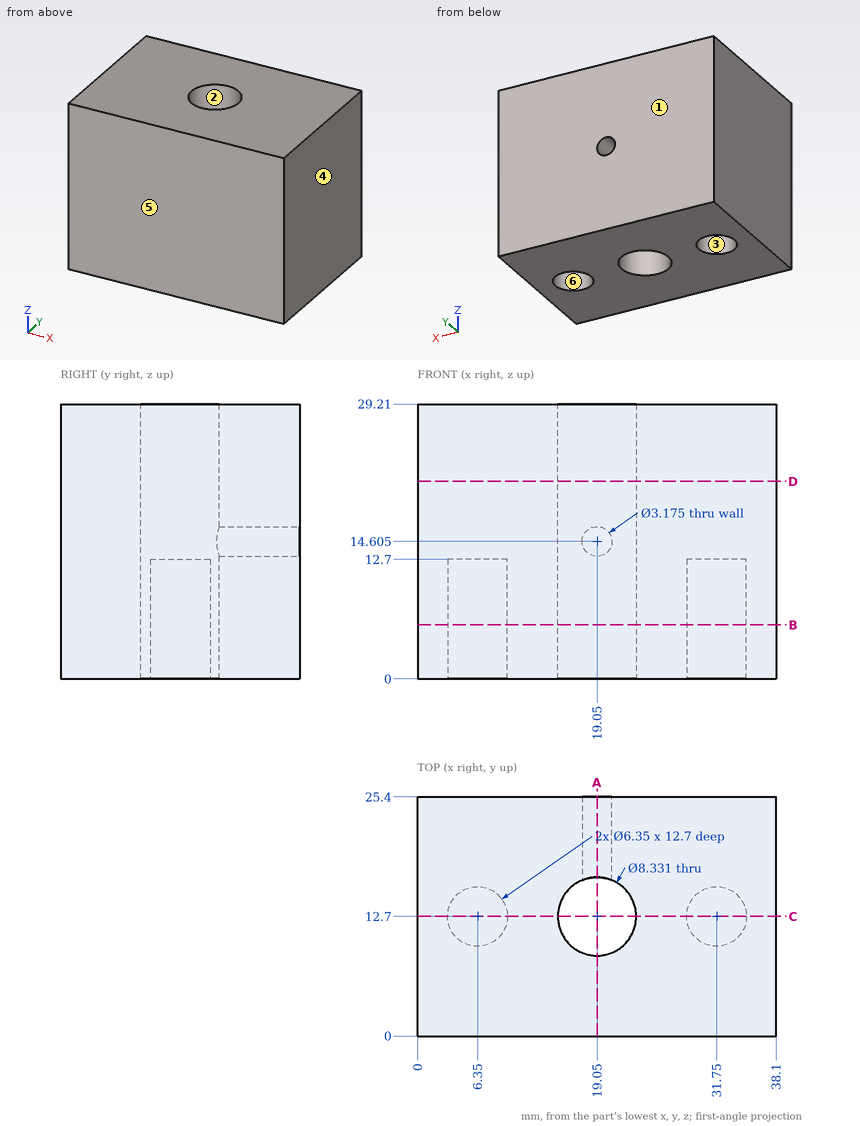
Print and shaded views of the part. All mm, measured from the part's lowest x, y and z. A direction names the side the tool comes from. Coordinates: 2 decimals unless noted, no trailing zeros. Write each loop counter-clockwise with the first axis right and the second up, starting at its lowest first coordinate (ties: lowest second). Pieces come first, ordered by that corner, then holes.
(1) Cut at D-D, the plane z = 21. List the corners of the cut face in (x, y), and give its area (3 significant figures).
(2) Cut at C-C, the plane y = 12.7. List the corners of the cut face in (x, z) (1 decimal), and give its area (3 significant figures).
(3) Drill centre lines: probe 1 along Y at (x, z) = (19.05, 23); probe 2 along X at (y, z) = (10.25, 10.25); probe 3 along Y at (x, z) = (31.75, 8.25) (3 decimals). Where is each one in solid material? Low to high.
(4) Flat gauge pin, fed straight in: pin 1 (1.9 mm diameter, centred on x = 7, y = 13, fed in from -Z). Where does the tip first touch, or does it go through?
(5) Cut at B-B, the plane z = 5.75. Count the separate pieces of the cut face and the enclosed holes in it, and give its area (3 significant figures).
(6) 3-axis set-ups, long thin cutter, end or side, ignore diameter. For the marked faces 5 and 6: which of +Z, -Z, +X, -X, +Y, -Y reach the whole face in a straight line?
(7) Cut at A-A, the plane x = 19.05. List the corners of the cut face in (y, z).
(8) Two-plate mould, pull along Y, no slides. Class the marked faces 1, 2, 3 and 4: +Y half, -Y half, draft (parallel to the pull), parting line (faces both ways), or undercut.
Geometry says:
1. outline: (0, 0) - (38.1, 0) - (38.1, 25.4) - (0, 25.4) - close; hole circle Ø8.33 at (19.05, 12.7)
1. area: 913 mm2
2. outline: (0, 0) - (3.2, 0) - (3.2, 12.7) - (9.5, 12.7) - (9.5, 0) - (14.9, 0) - (14.9, 29.2) - (0, 29.2) - close; (23.2, 0) - (28.6, 0) - (28.6, 12.7) - (34.9, 12.7) - (34.9, 0) - (38.1, 0) - (38.1, 29.2) - (23.2, 29.2) - close
2. area: 708 mm2
3. probe 1: y = 0 to 8.53, 16.87 to 25.4
3. probe 2: x = 0 to 4.33, 8.37 to 15.68, 22.42 to 29.73, 33.77 to 38.1
3. probe 3: y = 0 to 9.525, 15.875 to 25.4
4. pin 1: stops at z = 12.7
5. separate pieces: 1
5. enclosed holes: 3
5. area: 850 mm2
6. face 5: +Z, -Z, +X, -X, -Y
6. face 6: -Z
7. outline: (0, 0) - (8.53, 0) - (8.53, 29.21) - (0, 29.21) - close; (16.87, 0) - (25.4, 0) - (25.4, 13.02) - (16.87, 13.02) - close; (16.87, 16.19) - (25.4, 16.19) - (25.4, 29.21) - (16.87, 29.21) - close
8. face 1: +Y half
8. face 2: undercut
8. face 3: undercut
8. face 4: draft
